from build123d import *

# Parameters (mm, degrees)
F0_R          = 19.05
F1_DEPTH      = 127
F2_R          = 12.7
F3_DEPTH      = 12.7
F6_R          = 19.05
F7_DEPTH      = 76.2
F7_DEPTH_BACK = 76.2


with BuildPart() as f1:
    # F0 (on Top) → F1 (new body)
    with BuildSketch(Plane.XY):
        Circle(F0_R)
    extrude(amount=F1_DEPTH)

    # F2 (on face) → F3 (join)
    with BuildSketch(Plane(origin=(0, 0, 0), x_dir=(1, 0, 0), z_dir=(0, 0, -1))):
        Circle(F2_R)
    extrude(amount=F3_DEPTH)

    # F6 (on face) → F7 (join, two sides)
    with BuildSketch(Plane(origin=(0, 0, 0), x_dir=(-1, 0, 0), z_dir=(0, 1, 0))) as f7_sk:
        with Locations((0, 127)):
            Circle(F6_R)
    extrude(amount=F7_DEPTH)
    extrude(f7_sk.sketch, amount=-F7_DEPTH_BACK)


solid = f1.part
Part model, mm, in its own coordinate system. A direction names the side the tool comes from. Coordinates: 2 decimals unless noted, no trailing zeros. Loops run counter-clockwise (first coordinate to the right, second up) from the corner with the lowest first, then second, coordinate; pieces in that order, holes last. Notation, with made-up numbers: M 63.25,-22 L 92.25,-22 A16 cw 92.25,-12 Z; hole C 33,-5.5 d1. An arc over 180 degrees is marked long. Use a Markdown table: item, result. Add a question column.
Q1. Cut at D-D (z = 13). Write the cut outline in (x, y), and give its area (3 significant figures).
Q2. Probe L1, parallel to Y at x = -10.5, z = 98.5; L2, parallel to Z at x = -2, y = 55.5; L3, parallel to Y at x = -1, z = 66.5. List the from-to ranges inside material, lowest first.
Q3. Pin check, flat tips, straight feed: P1, Ø2, axis at y = -8, z = 102, coming from the +X side; P2, Ø3, axis at x = -13, z = 66.5, coming from the +Y side; P3, Ø2, axis at x = -5.5, y = -20, coming from the +Z side; P4, Ø10, axis at y = -29, z = 25, coming from the +X side. Stop position of each tip, or through.
Q4. Cut at A-A (x = 0). Write the cut outline in (y, z), and give its area (3 significant figures).
Q5. Which spindle directions (+Z, -Z, +X, -X, +Y, -Y) get a long thin tool onto all of the face, cutting with end or side? Do faces 1 (the flat face through (4, -12.4, 0)), 2 (the flat face through (0, -76.2, 127)). Say none if no direction does.
Q6. Cut at C-C (y = -57). Write the cut outline in (x, z), and give its area (3 significant figures).
Q7. Cut at B-B (z = 119). Write the cut outline in (x, y), and give its area (3 significant figures).
Worked out:
| question | item | result |
|---|---|---|
| 1 | outline | C 0,0 d38.1 |
| 1 | area | 1,140 mm2 |
| 2 | L1 | y = -15.9 to 15.9 |
| 2 | L2 | z = 108.06 to 145.94 |
| 2 | L3 | y = -19.02 to 19.02 |
| 3 | P1 | stops at x = 17.72 |
| 3 | P2 | stops at y = 15.19 |
| 3 | P3 | stops at z = 145.51 |
| 3 | P4 | passes through |
| 4 | outline | M -76.2,107.95 L -19.05,107.95 L -19.05,0 L -12.7,0 L -12.7,-12.7 L 12.7,-12.7 L 12.7,0 L 19.05,0 L 19.05,107.95 L 76.2,107.95 L 76.2,146.05 L -76.2,146.05 Z |
| 4 | area | 10,200 mm2 |
| 5 | face 1 | -Z |
| 5 | face 2 | +Z, -Z, +X, -X, -Y |
| 6 | outline | C 0,127 d38.1 |
| 6 | area | 1,140 mm2 |
| 7 | outline | M -17.29,-76.2 L 17.29,-76.2 L 17.29,-8 A19.05 ccw 17.29,8 L 17.29,76.2 L -17.29,76.2 L -17.29,8 A19.05 ccw -17.29,-8 Z |
| 7 | area | 5,310 mm2 |
